Build history of the part. All positions in model axes, mm. A direction names the side the tool comes from. Give positions to 0.01 mm unless a question says otherwise; leave off trailing zeros. Write each loop counter-clockwise with the first axis right and the second up, starting at its lowest first coordinate (ties: lowest second). Pieces come first, ordered by that corner, then holes. Notation, with made-up numbers: (21.5, -38) - (69.5, -38) arc R30 ccw to (69.5, -14) - close; hole circle Ø4 at (79, -33.5). An arc over 180 degrees is marked (long way). Use one line per item in the form item = value. Start each with the question number.
from build123d import *

# Parameters (mm, degrees)
DODANIE_WYCI_GNI_CIE1_DEPTH      = 108
DODANIE_WYCI_GNI_CIE1_DEPTH_BACK = 6
SZKIC1_W                         = 6
SZKIC1_H                         = 327
SZKIC2_W                         = 10
SZKIC2_H                         = 40
WYTNIJ_WYCI_GNI_CIE1_DEPTH       = 6
SZKIC7_R                         = 1.55
WYTNIJ_WYCI_GNI_CIE2_DEPTH       = 6
WYTNIJ_WYCI_GNI_CIE3_DEPTH       = 6
SZYK_LINIOWY1_COUNT              = 2
SZYK_LINIOWY1_PITCH              = 180
SZKIC9_W                         = 22
SZKIC9_H                         = 13
WYTNIJ_WYCI_GNI_CIE4_DEPTH       = 6
SZKIC11_R                        = 1.55
WYTNIJ_WYCI_GNI_CIE5_DEPTH       = 6
SZYK_LINIOWY2_COUNT              = 2
SZYK_LINIOWY2_PITCH              = 100
SZYK_LINIOWY2_COL_COUNT          = 2
SZYK_LINIOWY2_COL_PITCH          = 200
SZKIC14_R                        = 1.55
WYTNIJ_WYCI_GNI_CIE7_DEPTH       = 6
WYTNIJ_WYCI_GNI_CIE9_DEPTH       = 6


with BuildPart() as part:
    # Szkic1 → Dodanie-wyciągnięcie1 (new, two sides: drawn at the far end of the back side and taken through both)
    with BuildSketch(Plane.XY.offset(-DODANIE_WYCI_GNI_CIE1_DEPTH_BACK)):
        with Locations((-53, -253.103962956)):
            Rectangle(SZKIC1_W, SZKIC1_H)
    extrude(amount=DODANIE_WYCI_GNI_CIE1_DEPTH + DODANIE_WYCI_GNI_CIE1_DEPTH_BACK)

    # Szkic2 → Wytnij-wyciągnięcie1 (cut)
    with BuildSketch(Plane.ZY.offset(56)):
        with Locations((-1, -396.603962956)):
            Rectangle(SZKIC2_W, SZKIC2_H)
        with Locations((-1, -336.603962956)):
            Rectangle(SZKIC2_W, SZKIC2_H)
        Polygon((4, -176.603962956), (4, -42.619854706), (-6, -42.619854706), (-6, -176.603962956), (-6, -196.603962956), (-6, -236.603962956), (4, -236.603962956), (4, -196.603962956), align=None)
        with Locations((-1, -276.603962956)):
            Rectangle(SZKIC2_W, SZKIC2_H)
    extrude(amount=-WYTNIJ_WYCI_GNI_CIE1_DEPTH, mode=Mode.SUBTRACT)

    # Szkic7 → Wytnij-wyciągnięcie2 (cut)
    with BuildSketch(Plane.ZY.offset(56)):
        with Locations((57, -413.603962956)):
            Circle(SZKIC7_R)
    extrude(amount=-WYTNIJ_WYCI_GNI_CIE2_DEPTH, mode=Mode.SUBTRACT)

    # Szkic8 → Wytnij-wyciągnięcie3 (cut)
    with BuildSketch(Plane.ZY.offset(56)):
        Polygon((4, -395.053962956), (11, -395.053962956), (11, -393.678962956), (13, -393.678962956), (13, -395.053962956), (13.5, -395.053962956), (13.5, -398.153962956), (13, -398.153962956), (13, -399.528962956), (11, -399.528962956), (11, -398.153962956), (4, -398.153962956), align=None)
    wytnij_wyci_gni_cie3 = extrude(amount=-WYTNIJ_WYCI_GNI_CIE3_DEPTH, mode=Mode.SUBTRACT)

    # Szyk liniowy1: Wytnij-wyciągnięcie3 ×2
    with Locations(*[(0, i * SZYK_LINIOWY1_PITCH, 0) for i in range(1, SZYK_LINIOWY1_COUNT)]):
        add(wytnij_wyci_gni_cie3, mode=Mode.SUBTRACT)

    # Szkic9 → Wytnij-wyciągnięcie4 (cut)
    with BuildSketch(Plane.ZY.offset(56)):
        with Locations((65, -96.103962956)):
            Rectangle(SZKIC9_W, SZKIC9_H)
    extrude(amount=-WYTNIJ_WYCI_GNI_CIE4_DEPTH, mode=Mode.SUBTRACT)

    # Szkic11 → Wytnij-wyciągnięcie5 (cut)
    with BuildSketch(Plane.ZY.offset(56)):
        with Locations(Location((105, -386.603962956, 0), (0, 0, 270))):
            Circle(SZKIC11_R)
    wytnij_wyci_gni_cie5 = extrude(amount=-WYTNIJ_WYCI_GNI_CIE5_DEPTH, mode=Mode.SUBTRACT)

    # Szyk liniowy2: Wytnij-wyciągnięcie5 ×2
    with Locations(*[(0, i * SZYK_LINIOWY2_PITCH, 0) for i in range(1, SZYK_LINIOWY2_COUNT)]):
        add(wytnij_wyci_gni_cie5, mode=Mode.SUBTRACT)

    # Szyk liniowy2 col: Wytnij-wyciągnięcie5 ×2
    with Locations(*[(0, i * SZYK_LINIOWY2_COL_PITCH, 0) for i in range(1, SZYK_LINIOWY2_COL_COUNT)]):
        add(wytnij_wyci_gni_cie5, mode=Mode.SUBTRACT)

    # Szkic14 → Wytnij-wyciągnięcie7 (cut)
    with BuildSketch(Plane(origin=(-50, 0, 0), x_dir=(0, 0, -1), z_dir=(1, 0, 0))):
        with Locations(Location((-68, -376.603962956, 0), (0, 0, 90))):
            Circle(SZKIC14_R)
        with Locations(Location((-9.5, -232.603962956, 0), (0, 0, 90))):
            Circle(SZKIC14_R)
        with Locations(Location((-61.5, -232.603962956, 0), (0, 0, 90))):
            Circle(SZKIC14_R)
        with Locations(Location((-61.5, -344.603962956, 0), (0, 0, 90))):
            Circle(SZKIC14_R)
        with Locations(Location((-9.5, -344.603962956, 0), (0, 0, 90))):
            Circle(SZKIC14_R)
    extrude(amount=-WYTNIJ_WYCI_GNI_CIE7_DEPTH, mode=Mode.SUBTRACT)

    # Szkic15 → Wytnij-wyciągnięcie9 (cut)
    with BuildSketch(Plane.ZY.offset(56)):
        with BuildLine():
            Line((4, -172.624757885), (4, -89.603962956))
            Line((4, -89.603962956), (54, -89.603962956))
            Line((54, -89.603962956), (54, -102.603962956))
            Line((54, -102.603962956), (76, -102.603962956))
            Line((76, -102.603962956), (76, -89.603962956))
            Line((76, -89.603962956), (108, -89.603962956))
            Line((108, -89.603962956), (108, -163.601221201))
            ThreePointArc((108, -163.601221201), (56.219772668, -167.781476219), (4.492818283, -172.576125802))
            Line((4.492818283, -172.576125802), (4, -172.624757885))
        make_face()
    extrude(amount=-WYTNIJ_WYCI_GNI_CIE9_DEPTH, mode=Mode.SUBTRACT)


solid = part.part
(1) Cut at B-B, the plane y = -268. Give the cut face in (x, z), then the cut area to 3 significant figures.
(2) Cut at A-A, the plane x = -51. State how many separate pieces and enclosed holes the cut face has, then the cut area to 3 significant figures.
(3) Two-plate mould, pull along Y, no slides. Class faces 4 (the cylindrical face through (-53.04, -167.72, 56.94)), 5 (the flat face through (-53, -395.054, 7)), 6 (the flat face through (-53, -408, 4)): +Y half, -Y half, draft (parallel to the pull), parting line (faces both ways), or undercut.
(4) Pin check, flat tips, straight feed: pin 1 Ø1.8 at (x, y) = (-53, -187.5) entering from -Z; pin 2 Ø3 at (y, z) = (-232.6, 61.5) entering from -X; pin 3 Ø1.5 at (x, z) = (-53, 90.5) entering from +Y; pin 4 Ø3 at (x, z) = (-53.5, -3) entering from -Y. Stop position of each tip, or through.
(5) Wall check: line 1 (Y direction, x = -53.5, z = 2.5); line 2 (Z direction, x = -52.1, y = -233); line 3 (Z direction, x = -50.25, y = -346). Give the ranges that are in metal, low to high. Write a range as from..to.
(6) Cut at C-C, the plane z = 29.5. Give the cut face in (x, y).
(7) Which spindle directions (+Z, -Z, +X, -X, +Y, -Y) get a long thin tool onto all of the face, cutting with end or side? Do faces 1 (the flat face through (-53, -194, 4)), 2 (the flat face through (-53, -277, 4)), 3 (the flat face through (-53, -416.604, 55)). Say none if no direction does.
Solution:
q1.outline = (-56, 4) - (-50, 4) - (-50, 108) - (-56, 108) - close
q1.area = 624 mm2
q2.separate_pieces = 1
q2.enclosed_holes = 9
q2.area = 26,300 mm2
q3.face_4 = +Y half
q3.face_5 = undercut
q3.face_6 = draft
q4.pin_1 = 4
q4.pin_2 = through
q4.pin_3 = -164.89
q4.pin_4 = -376.6
q5.line_1 = -376.6..-356.6, -316.6..-296.6, -256.6..-236.6
q5.line_2 = 4..8, 11..60, 63..108
q5.line_3 = 4..8.83, 10.17..60.83, 62.17..108
q6.outline = (-56, -416.6) - (-50, -416.6) - (-50, -170.18) - (-56, -170.18) - close
q7.face_1 = -Z, +X, -X, +Y
q7.face_2 = -Z, +X, -X
q7.face_3 = +Z, -Z, +X, -X, -Y
